Drawing for the job (mm, zero at the part's lowest x, y, z). Give positions to 0.01 mm unless a question says otherwise; leave off trailing zeros. Order: outer loops, then holes, each group sorted by start corner. A loop starts at its lowest first (then second) coordinate and runs counter-clockwise, first axis right, second up. Notation, with made-up numbers: (69.25, 26.25) -> (116.25, 26.25) arc R23 ccw to (116.25, 48.25) -> close; hole circle Ø6 at (39, 67). An arc over 180 degrees is marked (long way). Use a Markdown table: item, result. Add a question column.
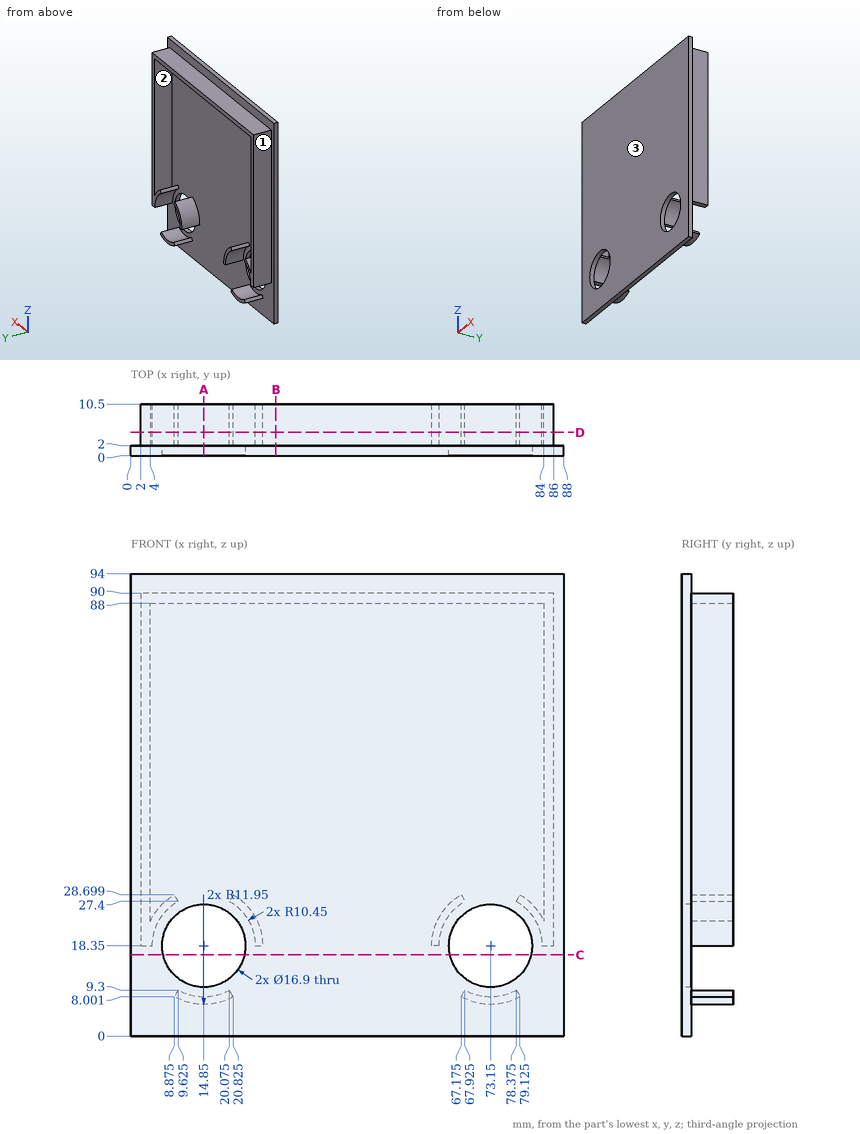
(1) Wall check: probe 1 along Z at (x, y) = (14.85, 0.7); probe 2 along X at (y, z) = (9, 86.5); probe 3 along Z at (x, y) = (14.5, 4.75). Give the ranges that are in metal, low to high.
(2) Band-saw the part on A-A on x = 14.85. Give the cut face in (y, z).
(3) Band-saw the part on D-D on y = 4.75. State how many separate pieces and enclosed holes the cut face has, plus the area to 3 significant figures.
(4) Pin check, flat tips, straight feed: pin 1 Ø1.2 at (x, y) = (26, 8) entering from -Z; pin 2 Ø2 at (x, y) = (16.5, 8) entering from +Z; pin 3 Ø4 at (x, y) = (36.5, 4.5) entering from -Z; pin 4 Ø10 at (x, z) = (73.15, 18.35) entering from -Y. Stop position of each tip, or through.
(5) Band-saw the part on B-B on x = 29.5. Give the cut face in (y, z).
(6) Mould opens along X. For the marked faces 1, 2 and 3 say: released by +X, released by -X, zero draft, split by the parting line, or undercut.
(7) Band-saw the part on C-C on z = 16.5. Give the cut face in (x, y) (3 decimals), plus the area to 3 significant figures.
Response:
| question | item | result |
|---|---|---|
| 1 | probe 1 | z = 0 to 9.9, 26.8 to 94 |
| 1 | probe 2 | x = 2 to 4, 84 to 86 |
| 1 | probe 3 | z = 6.41 to 7.91, 88 to 90 |
| 2 | outline | (0, 0) -> (2, 0) -> (2, 6.4) -> (10.5, 6.4) -> (10.5, 7.9) -> (2, 7.9) -> (2, 9.9) -> (0, 9.9) -> close; (0, 26.8) -> (2, 26.8) -> (2, 88) -> (10.5, 88) -> (10.5, 90) -> (2, 90) -> (2, 94) -> (0, 94) -> close |
| 3 | separate pieces | 5 |
| 3 | enclosed holes | 0 |
| 3 | area | 545 mm² |
| 4 | pin 1 | stops at z = 18.35 |
| 4 | pin 2 | stops at z = 90 |
| 4 | pin 3 | stops at z = 88 |
| 4 | pin 4 | passes through |
| 5 | outline | (0, 0) -> (2, 0) -> (2, 88) -> (10.5, 88) -> (10.5, 90) -> (2, 90) -> (2, 94) -> (0, 94) -> close |
| 6 | face 1 | released by -X |
| 6 | face 2 | undercut |
| 6 | face 3 | zero draft |
| 7 | outline | (0, 0) -> (6.605, 0) -> (6.605, 2) -> (0, 2) -> close; (23.095, 0) -> (64.905, 0) -> (64.905, 2) -> (23.095, 2) -> close; (81.395, 0) -> (88, 0) -> (88, 2) -> (81.395, 2) -> close |
| 7 | area | 110 mm² |
